Source: CAD feature listing. Evaluate the final solid. Frame: model axes, mm. A direction names the side the tool comes from. Round coordinates to 2 decimals unless told otherwise and drop trailing zeros. Loops run counter-clockwise (first coordinate to the right, second up) from the corner with the lowest first, then second, coordinate; pieces in that order, holes last. Notation, with made-up numbers: (52, 45) -> (97, 45) arc R27 cw to (97, 66) -> close; hole circle Ø11 at (-9.5, 13). An arc over 180 degrees is marked (long way). Return JSON: item names as keys, results as strings. Group by question number.
```python
from build123d import *

# Parameters (mm, degrees)
CROQUIS4_W                = 13
CROQUIS4_H                = 11.3
SALIENTE_EXTRUIR1_DEPTH   = 161
CROQUIS5_W                = 151
CROQUIS5_H                = 3.5
CORTAR_EXTRUIR1_DEPTH     = 6.3
SALIENTE_EXTRUIR3_DEPTH   = 8
CROQUIS9_R                = 2.5
CORTAR_EXTRUIR3_DEPTH     = 179.518038304
SIMETR_A8_COPY_1_DEPTH    = 8
SIMETR_A8_COPY_2_SKETCH_R = 2.5
SIMETR_A8_COPY_2_DEPTH    = 179.518038304
CROQUIS10_R               = 2.5
CORTAR_EXTRUIR4_DEPTH     = 179.518038304
MATRIZL1_COUNT            = 3
MATRIZL1_PITCH            = 40.5
CROQUIS11_W               = 64.853728184
CROQUIS11_H               = 22.965019475
CORTAR_EXTRUIR5_DEPTH     = 167.107465215
CROQUIS12_W               = 8
CROQUIS12_H               = 6.3
CORTAR_EXTRUIR6_DEPTH     = 45.010680522


with BuildPart() as part:
    # Barrer1: sweep along a path in Croquis3
    with BuildLine(Plane(origin=(0, 0, 0), x_dir=(1, 0, 0), z_dir=(0, 1, 0))) as barrer1_path:
        Line((0, 0), (0, -37))
    # Croquis1 → Barrer1 (sweep)
    with BuildSketch(Plane.XY):
        Polygon((0, 0), (0, 11.3), (13, 11.3), (13, 6.3), (5, 6.3), (5, 0), align=None)
    barrer1 = sweep(path=barrer1_path.line)

    # Croquis4 → Saliente-Extruir1 (add)
    with BuildSketch(Plane.ZY):
        with Locations((43.5, 5.65)):
            Rectangle(CROQUIS4_W, CROQUIS4_H)
    extrude(amount=-SALIENTE_EXTRUIR1_DEPTH)

    # Simetría5: Barrer1 across plane
    add(barrer1.mirror(Plane.ZY.offset(-80.5)))

    # Croquis5 → Cortar-Extruir1 (cut)
    with BuildSketch(Plane.XZ):
        with Locations((80.5, 38.75)):
            Rectangle(CROQUIS5_W, CROQUIS5_H)
    extrude(amount=-CORTAR_EXTRUIR1_DEPTH, mode=Mode.SUBTRACT)

    # Croquis8 → Saliente-Extruir3 (add)
    with BuildSketch(Plane.XZ):
        with BuildLine():
            Line((161, 47), (165, 47))
            ThreePointArc((165, 47), (171, 41), (165, 35))
            Line((165, 35), (161, 35))
            Line((161, 35), (161, 47))
        make_face()
    saliente_extruir3 = extrude(amount=-SALIENTE_EXTRUIR3_DEPTH)

    # Croquis9 → Cortar-Extruir3 (cut, through all)
    with BuildSketch(Plane.XZ):
        with Locations((165, 41)):
            Circle(CROQUIS9_R)
    cortar_extruir3 = extrude(amount=-CORTAR_EXTRUIR3_DEPTH, mode=Mode.SUBTRACT)

    # Simetría7: Saliente-Extruir3, Cortar-Extruir3 across plane
    add(saliente_extruir3.mirror(Plane(origin=(0, 0, 25), x_dir=(1, 0, 0), z_dir=(0, 0, -1))))
    add(cortar_extruir3.mirror(Plane(origin=(0, 0, 25), x_dir=(1, 0, 0), z_dir=(0, 0, -1))), mode=Mode.SUBTRACT)

    # Simetría8: Saliente-Extruir3, Cortar-Extruir3 across plane
    add(saliente_extruir3.mirror(Plane.ZY.offset(-80.5)))
    add(cortar_extruir3.mirror(Plane.ZY.offset(-80.5)), mode=Mode.SUBTRACT)

    # Simetría8 copy 1 sketch → Simetría8 copy 1 (add)
    with BuildSketch(Plane(origin=(161, 0, 50), x_dir=(-1, 0, 0), z_dir=(0, -1, 0))):
        with BuildLine():
            Line((161, 47), (165, 47))
            ThreePointArc((165, 47), (171, 41), (165, 35))
            Line((165, 35), (161, 35))
            Line((161, 35), (161, 47))
        make_face()
    extrude(amount=-SIMETR_A8_COPY_1_DEPTH)

    # Simetría8 copy 2 sketch → Simetría8 copy 2 (cut, through all)
    with BuildSketch(Plane(origin=(161, 0, 50), x_dir=(-1, 0, 0), z_dir=(0, -1, 0))):
        with Locations((165, 41)):
            Circle(SIMETR_A8_COPY_2_SKETCH_R)
    extrude(amount=-SIMETR_A8_COPY_2_DEPTH, mode=Mode.SUBTRACT)

    # Croquis10 → Cortar-Extruir4 (cut, through all)
    with BuildSketch(Plane(origin=(0, 11.3, 0), x_dir=(1, 0, 0), z_dir=(0, 1, 0))):
        with Locations(Location((121, -45.25, 0), (0, 0, 270))):
            Circle(CROQUIS10_R)
    cortar_extruir4 = extrude(amount=-CORTAR_EXTRUIR4_DEPTH, mode=Mode.SUBTRACT)

    # MatrizL1: Cortar-Extruir4 ×3
    with Locations(*[(-i * MATRIZL1_PITCH, 0, 0) for i in range(1, MATRIZL1_COUNT)]):
        add(cortar_extruir4, mode=Mode.SUBTRACT)

    # Croquis11 → Cortar-Extruir5 (cut, through all)
    with BuildSketch(Plane(origin=(13, 0, 0), x_dir=(0, 0, -1), z_dir=(1, 0, 0))):
        with Locations((-26.956517022, 7.895183468)):
            Rectangle(CROQUIS11_W, CROQUIS11_H)
    extrude(amount=CORTAR_EXTRUIR5_DEPTH, mode=Mode.SUBTRACT)

    # Croquis12 → Cortar-Extruir6 (cut, through all)
    with BuildSketch(Plane(origin=(0, 0, 40.5), x_dir=(-1, 0, 0), z_dir=(0, 0, -1))):
        with Locations((-9, 3.15)):
            Rectangle(CROQUIS12_W, CROQUIS12_H)
    extrude(amount=-CORTAR_EXTRUIR6_DEPTH, mode=Mode.SUBTRACT)


solid = part.part
```
(1) Cut plane D-D (z = 26). Return loops of the section in (x, y).
(2) Pin query (flat end, axial travel): pin 1 (5 mm diameter, centred on x = -5, z = 9, fed in from +Y); pin 2 (4 mm diameter, centred on y = 5.5, z = 37.5, fed in from -X); pin 3 (2 mm diameter, centred on x = -2.5, y = 4, fed in from +Z); pin 4 (3 mm diameter, centred on x = -4, z = 9, fed in from +Y). Return the tip coordinate at first contact, or that it passes through.
(3) Cut plane C-C (y = 5). Return loops of the section in (x, z), and give its area (3 significant figures).
(4) Ray query, line 1 (Z direction, x = -4, y = 5); line 2 (X direction, y = 3.75, z = 41); line 3 (Z direction, x = -5, y = 5.5). Return the intervals inside material, ascending.
(5) Mould query, pull axis Z, two halves, no side actions, for faces 5 (the face through (-5, 8, 12)), 6 (the face through (-3.46, 3.94, 11.44)), 7 (the face through (-2, 4, 47)), 8 (the face through (0, 7, 25)). Classes: released by +Z, released by -Z, zero draft, split by the parting line, or undercut.
(6) Cut plane B-B (x = -2.75). Return loops of the section in (y, z).
(7) Set-up query: faces 1 (the face through (-2, 4, 3)), 2 (the face through (-2, 4, 35)), 3 (the face through (9, 6.3, 25)), 4 (the face through (-5, 8, 38)). Return all of +Z, -Z, +X, -X, +Y, -Y with unobstructed straight access to the full face (end or side cutting, diameter ignored); none if empty.
(8) Cut plane A-A (z = 41). Return loops of the section in (x, y), and give its area (4 significant figures).
Answers follow:
{
 "1": {"outline": "(0, 0) -> (5, 0) -> (5, 6.3) -> (13, 6.3) -> (13, 11.3) -> (0, 11.3) -> close"},
 "2": {"pin 1": "y = 8", "pin 2": "x = -9.81", "pin 3": "z = 47", "pin 4": "through"},
 "3": {"outline": "(-4, 3) -> (0, 3) -> (0, 0) -> (5, 0) -> (5, 50) -> (0, 50) -> (0, 47) -> (-4, 47) arc R6 ccw to (-4, 35) -> (0, 35) -> (0, 15) -> (-4, 15) arc R6 ccw to start; hole circle Ø5 at (-4, 9); hole circle Ø5 at (-4, 41)", "area": "420 mm^2"},
 "4": {"line 1": "3 to 6.5, 11.5 to 15, 35 to 38.5, 43.5 to 47", "line 2": "-10 to -6.5, -1.5 to 5", "line 3": "3.08 to 6.71, 11.29 to 14.92, 35.08 to 38.71, 43.29 to 46.92"},
 "5": {"face 5": "zero draft", "face 6": "undercut", "face 7": "released by +Z", "face 8": "undercut"},
 "6": {"outline": "(0, 3) -> (8, 3) -> (8, 6.83) -> (0, 6.83) -> close; (0, 11.17) -> (8, 11.17) -> (8, 15) -> (0, 15) -> close; (0, 35) -> (8, 35) -> (8, 38.83) -> (0, 38.83) -> close; (0, 43.17) -> (8, 43.17) -> (8, 47) -> (0, 47) -> close"},
 "7": {"face 1": "-Z, -X, +Y, -Y", "face 2": "-X, +Y, -Y", "face 3": "+Z, -Z, +X, -Y", "face 4": "+Z, -Z, -X, +Y"},
 "8": {"outline": "(-10, 0) -> (-6.5, 0) -> (-6.5, 8) -> (-10, 8) -> close; (-1.5, 0) -> (5, 0) -> (5, 6.3) -> (13, 6.3) -> (13, 11.3) -> (0, 11.3) -> (0, 8) -> (-1.5, 8) -> close", "area": "136.5 mm^2"}
}
